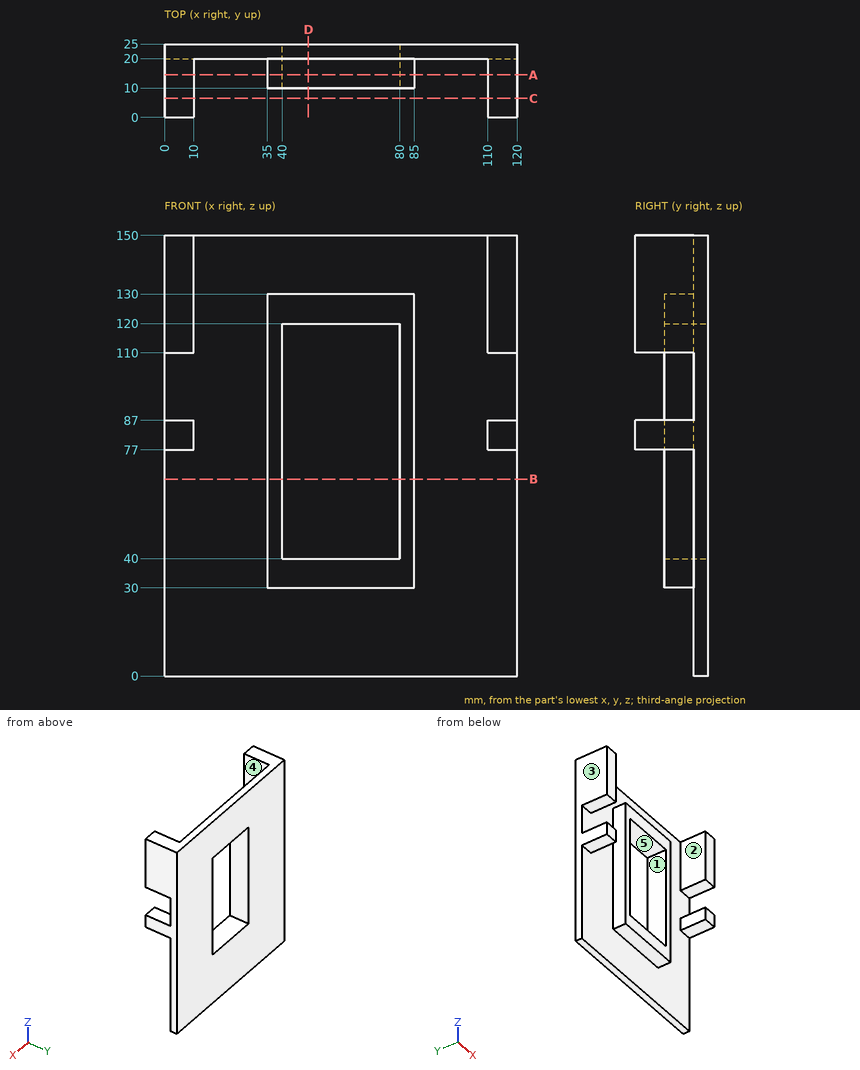
Source: three-view drawing plus pictorial views. Frame: mm from the lowest corner of the part. A direction names the side the tool comes from. Round coordinates to 2 decimals unless told otherwise and drop trailing zeros. Write each loop counter-clockwise with the first axis right and the second up, starting at its lowest first coordinate (ties: lowest second). Pieces come first, ordered by that corner, then holes. Notation, with made-up numbers: M 46.5,33 L 95.5,33 A21 ccw 95.5,62 Z; hole C -16,-37.5 d10. An arc over 180 degrees is marked long. Use CSV: the item, a comma, the result in double quotes. Start each with the question number.
Q1. First-contact query: P1, Ø3, axis at x = 114, y = 9.5, coming from the -Z side; P2, Ø4.5, axis at x = 63, y = 15.5, coming from the +Z side; P3, Ø1, axis at x = 100.5, z = 27.5, coming from the -Y side. Flat tips, straight axial feed; report the tip coordinate or a pass-through.
Q2. Cut plane C-C on y = 6.5. Output: boundary loops of the cut face in (x, z), plus the area to 3 significant figures.
Q3. Cut plane B-B on z = 67. Output: boundary loops of the cut face in (x, y), plus the area to 3 significant figures.
Q4. Cut plane A-A on y = 14.5. Output: boundary loops of the cut face in (x, z).
Q5. Access query for the marked faces 3, 4 and 5. Directions: +Z, -Z, +X, -X, +Y, -Y. A direction counts if a zero-diameter tool reaches every point of the face in a straight line with its end or side. Return the directions, or none.
Q6. Pull-direction query (Z, two-part tool) for the marked faces 1 and 2; classes: +Z half, -Z half, draft (parallel to the pull), parting line (faces both ways), or undercut.
Q7. Cut plane D-D on x = 49. Output: boundary loops of the cut face in (y, z).
Q8. Line query: line 1 (X direction, y = 15, z = 79); line 2 (X direction, y = 18.5, z = 121); line 3 (Z direction, x = 62, y = 17.25). Output: solid intervals per line, ascending. Write a range as from..to.
Results found:
1,P1,"z = 77"
1,P2,"z = 130"
1,P3,"y = 20"
2,outline,"M 0,77 L 10,77 L 10,87 L 0,87 Z; M 0,110 L 10,110 L 10,150 L 0,150 Z; M 110,77 L 120,77 L 120,87 L 110,87 Z; M 110,110 L 120,110 L 120,150 L 110,150 Z"
2,area,"1,000 mm^2"
3,outline,"M 0,20 L 35,20 L 35,10 L 40,10 L 40,25 L 0,25 Z; M 80,10 L 85,10 L 85,20 L 120,20 L 120,25 L 80,25 Z"
3,area,"500 mm^2"
4,outline,"M 0,77 L 10,77 L 10,87 L 0,87 Z; M 0,110 L 10,110 L 10,150 L 0,150 Z; M 35,30 L 85,30 L 85,130 L 35,130 Z; M 110,77 L 120,77 L 120,87 L 110,87 Z; M 110,110 L 120,110 L 120,150 L 110,150 Z; hole M 40,40 L 80,40 L 80,120 L 40,120 Z"
5,face 3,"+Z, -Z, -X, +Y, -Y"
5,face 4,"+Z, -Z, -Y"
5,face 5,"+Y, -Y"
6,face 1,"undercut"
6,face 2,"draft"
7,outline,"M 10,30 L 20,30 L 20,0 L 25,0 L 25,40 L 10,40 Z; M 10,120 L 25,120 L 25,150 L 20,150 L 20,130 L 10,130 Z"
8,line 1,"0..10, 35..40, 80..85, 110..120"
8,line 2,"0..10, 35..85, 110..120"
8,line 3,"30..40, 120..130"
